```python
from build123d import *

# Parameters (mm, degrees)
SKETCH033_R             = 24.5
PAD011_DEPTH            = 29
SKETCH034_R             = 7.5
SKETCH034_R_2           = 1.5
PAD012_DEPTH            = 1
PAD013_DEPTH            = 38
BODY012_PLACEMENT_ANGLE = 90


with BuildPart() as part:
    # Sketch033 → Pad011 (new body)
    with BuildSketch(Plane.XY):
        Circle(SKETCH033_R)
    extrude(amount=-PAD011_DEPTH)

    # Sketch034 (on Face2 of Pad011) → Pad012 (join)
    with BuildSketch(Plane.XY):
        with BuildLine():
            Line((-31.107801, 2.74676), (-17.810284, 16.823905))
            ThreePointArc((17.810283, 16.823906), (-1e-06, 24.5), (-17.810284, 16.823905))
            Line((17.810283, 16.823906), (31.107801, 2.74676))
            ThreePointArc((31.107801, -2.74676), (32.2, 0), (31.107801, 2.74676))
            Line((17.810284, -16.823905), (31.107801, -2.74676))
            ThreePointArc((-17.810283, -16.823906), (1e-06, -24.5), (17.810284, -16.823905))
            Line((-31.107801, -2.74676), (-17.810283, -16.823906))
            ThreePointArc((-31.107801, 2.74676), (-32.2, 0), (-31.107801, -2.74676))
        make_face()
        Circle(SKETCH034_R, mode=Mode.SUBTRACT)
        with Locations((-28.2, 0)):
            Circle(SKETCH034_R_2, mode=Mode.SUBTRACT)
        with Locations((28.2, 0)):
            Circle(SKETCH034_R_2, mode=Mode.SUBTRACT)
    extrude(amount=PAD012_DEPTH)

    # Sketch035 (on Face17 of Pad012) → Pad013 (join)
    with BuildSketch(Plane.XY):
        Polygon((3.5, -6.062178), (7, 0), (3.5, 6.062178), (-3.5, 6.062178), (-7, 0), (-3.5, -6.062178), align=None)
    extrude(amount=PAD013_DEPTH)


with BuildPart() as part_1:
    # Body012 placement: moved
    add(part.part.moved(Location((48, 100, 48.5))).rotate(Axis((48, 100, 48.5), (0, 0, -1)), BODY012_PLACEMENT_ANGLE))


solid = part_1.part
```
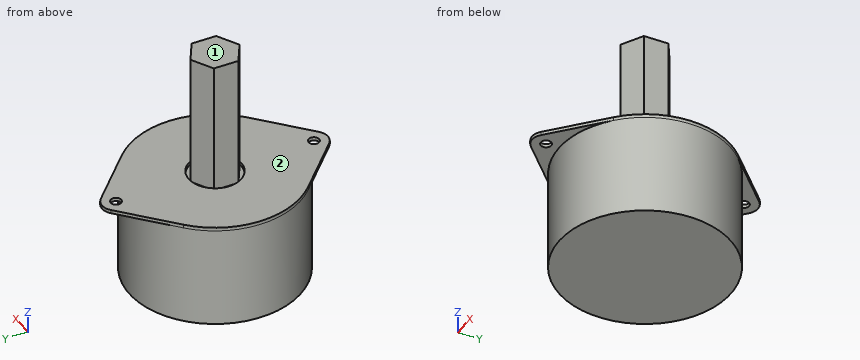
Geometry check sheet. Reference: the model listing, model coordinates, mm. Face numbers are marked on the shaded views. A direction names the side the tool comes from. Coordinates: 2 decimals unless noted, no trailing zeros. Order: outer loops, then holes, each group sorted by start corner. A loop starts at its lowest first (then second) coordinate and runs counter-clockwise, first axis right, second up. Notation, with made-up numbers: (61.5, -39.5) - (77.5, -39.5) arc R29 ccw to (77.5, -9.5) - close; hole circle Ø6 at (47.25, 60). An arc over 180 degrees is marked (long way). Answer as a JSON object with one key per item and string values. Group by question number.
Item 1: Sectioned sample at B-B, the plane z = 72.5. Record the cut outline in (x, y).
Item 2: Scan lines: probe 1 along X at (y, z) = (100, 49.15); probe 2 along Z at (x, y) = (55, 118); probe 3 along Z at (x, y) = (38, 122.5). Record each from-to range of solid material in increasing order.
Item 3: Sectioned sample at C-C, the plane y = 71.8. Record the cut outline in (x, z).
Item 4: Sectioned sample at A-A, the plane y = 100. Record the cut outline in (x, z).
Item 5: Sectioned sample at D-D, the plane x = 58.5. Record the cut outline in (y, z), and give its area (3 significant figures).
Item 6: Tool access check on the marked faces 1 and 2. Record the directions out of +Z, -Z, +X, -X, +Y, -Y that give a thin tool (end or side, any length) a straight path to the whole face; none if there is none.
Item 7: Depth check by flat-ended pin: pin 1 Ø4 at (x, y) = (48, 128.2) entering from +Z; pin 2 Ø5 at (x, z) = (30.5, 26.5) entering from -Y; pin 3 Ø1.5 at (y, z) = (98, 31.5) entering from -X. Enter the tip coordinate at first touch or a pass-through.
Resolved:
{
 "1": {"outline": "(41.94, 96.5) - (48, 93) - (54.06, 96.5) - (54.06, 103.5) - (48, 107) - (41.94, 103.5) - close"},
 "2": {"probe 1": "23.5 to 40.5, 41.94 to 54.06, 55.5 to 72.5", "probe 2": "19.5 to 49.5", "probe 3": "48.5 to 49.5"},
 "3": {"outline": "(42.17, 48.5) - (46.5, 48.5) - (46.5, 49.5) - (42.17, 49.5) - close; (49.5, 48.5) - (53.83, 48.5) - (53.83, 49.5) - (49.5, 49.5) - close"},
 "4": {"outline": "(23.5, 19.5) - (72.5, 19.5) - (72.5, 49.5) - (55.5, 49.5) - (55.5, 48.5) - (54.06, 48.5) - (54.06, 86.5) - (41.94, 86.5) - (41.94, 48.5) - (40.5, 48.5) - (40.5, 49.5) - (23.5, 49.5) - close"},
 "5": {"outline": "(76.22, 48.5) - (77.86, 48.5) - (77.86, 19.5) - (122.14, 19.5) - (122.14, 48.5) - (123.78, 48.5) - (123.78, 49.5) - (76.22, 49.5) - close", "area": "1,330 mm^2"},
 "6": {"face 1": "+Z, +X, -X, +Y, -Y", "face 2": "+Z"},
 "7": {"pin 1": "z = 49.5", "pin 2": "y = 80.63", "pin 3": "x = 23.53"}
}
